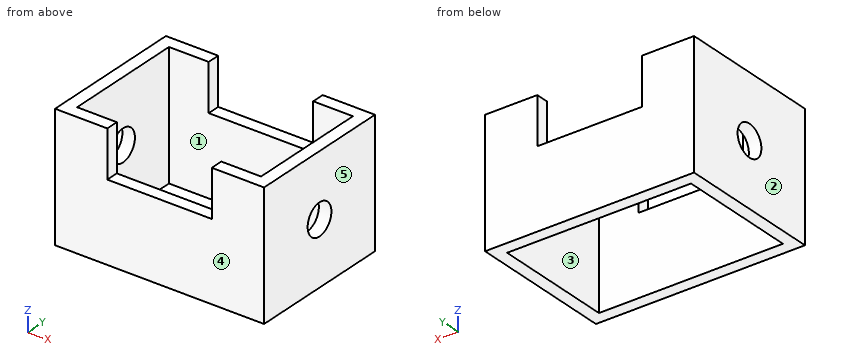
```python
from build123d import *

# Parameters (mm, degrees)
F0_W     = 200
F0_H     = 140
F0_W_2   = 176
F0_H_2   = 116
F1_DEPTH = 120
F2_R     = 15
F3_DEPTH = 200.001
F4_W     = 100
F4_H     = 45
F5_DEPTH = 140.001


with BuildPart() as f1:
    # F0 (on Top) → F1 (new body)
    with BuildSketch(Plane.XY):
        Rectangle(F0_W, F0_H)
        Rectangle(F0_W_2, F0_H_2, mode=Mode.SUBTRACT)
    extrude(amount=F1_DEPTH)

    # F2 (on face) → F3 (cut, through all)
    with BuildSketch(Plane.YZ.offset(100)):
        with Locations((0, 60)):
            Circle(F2_R)
    extrude(amount=-F3_DEPTH, mode=Mode.SUBTRACT)

    # F4 (on face) → F5 (cut, through all)
    with BuildSketch(Plane.XZ.offset(70)):
        with Locations((0, 97.5)):
            Rectangle(F4_W, F4_H)
    extrude(amount=-F5_DEPTH, mode=Mode.SUBTRACT)


solid = f1.part
```
CAD build for the part. Positions are in the model's coordinates, mm. Face numbers are marked on the shaded views. A direction names the side the tool comes from. Coordinates: 2 decimals unless noted, no trailing zeros. Write each loop counter-clockwise with the first axis right and the second up, starting at its lowest first coordinate (ties: lowest second). Pieces come first, ordered by that corner, then holes. Notation, with made-up numbers: (42.25, -33) -> (48.25, -33) arc R16 cw to (48.25, -4) -> close; hole circle Ø5 at (2.5, -29.75). An arc over 180 degrees is marked (long way). Use CSV: the item, a comma, the result in double quotes. Start each with the question number.
Item 1: Wall check: probe 1 along Z at (x, y) = (-96, 0); probe 2 along X at (y, z) = (-50, 66); probe 3 along Y at (x, z) = (-14.5, 74). Give the ranges that are in metal, low to high.
Item 2: Two-plate mould, pull along Y, no slides. Class the marked faces 3, 4 and 5: +Y half, -Y half, draft (parallel to the pull), parting line (faces both ways), or undercut.
Item 3: Band-saw the part on A-A, the plane z = 80.5. Write the cut outline in (x, y).
Item 4: Band-saw the part on D-D, the plane z = 17.5. Write the cut outline in (x, y), plus the area to 3 significant figures.
Item 5: Tool access for the marked faces 1 and 2: list every direction of +Z, -Z, +X, -X, +Y, -Y with a clear straight run to the whole face (end or side of a thin tool).
Item 6: Band-saw the part on C-C, the plane y = -43.5. Write the cut outline in (x, z).
Item 7: Drop a flat-ended pin along its axis: P1, Ø13, axis at x = -5, y = 63.5, coming from the +Z side. Give the stop position or say it passes through.
Item 8: Band-saw the part on B-B, the plane x = 66.5. Write the cut outline in (y, z).
Response values:
1,probe 1,"z = 0 to 45, 75 to 120"
1,probe 2,"x = -100 to -88, 88 to 100"
1,probe 3,"y = -70 to -58, 58 to 70"
2,face 3,"undercut"
2,face 4,"-Y half"
2,face 5,"draft"
3,outline,"(-100, -70) -> (-50, -70) -> (-50, -58) -> (-88, -58) -> (-88, 58) -> (-50, 58) -> (-50, 70) -> (-100, 70) -> close; (50, -70) -> (100, -70) -> (100, 70) -> (50, 70) -> (50, 58) -> (88, 58) -> (88, -58) -> (50, -58) -> close"
4,outline,"(-100, -70) -> (100, -70) -> (100, 70) -> (-100, 70) -> close; hole (-88, -58) -> (88, -58) -> (88, 58) -> (-88, 58) -> close"
4,area,"7,580 mm2"
5,face 1,"+Z, -Z"
5,face 2,"+Z, -Z, -X, +Y, -Y"
6,outline,"(-100, 0) -> (-88, 0) -> (-88, 120) -> (-100, 120) -> close; (88, 0) -> (100, 0) -> (100, 120) -> (88, 120) -> close"
7,P1,"stops at z = 75"
8,outline,"(-70, 0) -> (-58, 0) -> (-58, 120) -> (-70, 120) -> close; (58, 0) -> (70, 0) -> (70, 120) -> (58, 120) -> close"
